```python
from build123d import *

# Parameters (mm, degrees)
SKETCH_3_R               = 7.5
CUT_EXTRUDE_1_DEPTH      = 342.0278581
SKETCH_4_R               = 35
CUT_EXTRUDE_2_DEPTH      = 342.0278581
SWEEP_2_PROFILE_R        = 5.5
CUT_EXTRUDE_4_DEPTH      = 20
PATTERN_CIRCULAR_2_COUNT = 5


with BuildPart() as part:
    # Sketch 1 → Revolve 1 (revolve)
    with BuildSketch(Plane(origin=(0, 0, 0), x_dir=(1, 0, 0), z_dir=(0, 1, 0)), mode=Mode.PRIVATE) as revolve_1_sk:
        Polygon((170, 0), (190, 0), (190, -12), (176, -12), (176, -188), (190, -188), (190, -200), (170, -200), align=None)
    revolve(revolve_1_sk.sketch.rotate(Axis((0, 0, 0), (0, 0, 1)), 180), axis=Axis((0, 0, 0), (0, 0, 1)))

    # Sketch 2 → Revolve 2 (revolve)
    with BuildSketch(Plane(origin=(0, 0, 0), x_dir=(1, 0, 0), z_dir=(0, 1, 0)), mode=Mode.PRIVATE) as revolve_2_sk:
        Polygon((0, -140), (60, -140), (60, -150), (171, -150), (171, -170), (60, -170), (60, -210), (0, -210), align=None)
    revolve(revolve_2_sk.sketch.rotate(Axis((0, 0, 140), (0, 0, 1)), 180), axis=Axis((0, 0, 140), (0, 0, 1)))

    # Sketch 3 → Cut-Extrude 1 (cut, through all)
    with BuildSketch(Plane.XY.offset(210)):
        with Locations(Location((0, 57.15, 0), (0, 0, 18.896417832))):
            Circle(SKETCH_3_R)
        with Locations(Location((-54.35288, 17.660321, 0), (0, 0, 90.896417923))):
            Circle(SKETCH_3_R)
        with Locations(Location((-33.591927, -46.235321, 0), (0, 0, 305.10357978))):
            Circle(SKETCH_3_R)
        with Locations(Location((33.591927, -46.235321, 0), (0, 0, 17.103579776))):
            Circle(SKETCH_3_R)
        with Locations(Location((54.35288, 17.660321, 0), (0, 0, 306.896417429))):
            Circle(SKETCH_3_R)
    extrude(amount=-CUT_EXTRUDE_1_DEPTH, mode=Mode.SUBTRACT)

    # Sketch 4 → Cut-Extrude 2 (cut, through all)
    with BuildSketch(Plane.XY.offset(210)):
        Circle(SKETCH_4_R)
    extrude(amount=-CUT_EXTRUDE_2_DEPTH, mode=Mode.SUBTRACT)

    # Sweep 2: sweep along a curve in space
    with BuildLine() as sweep_2_path:
        Line((94.046, 129.443, 100), (124.876, 171.912, 100))
    # Sweep 2 profile (on start of the path) → Sweep 2 (sweep, cut)
    with BuildSketch(Plane(origin=(94.046, 129.443, 100), x_dir=(0.8092483062128621, -0.5874667470517917, 0), z_dir=(0.5874667470517917, 0.8092483062128621, 0))):
        Circle(SWEEP_2_PROFILE_R)
    sweep(path=sweep_2_path.line, mode=Mode.SUBTRACT)

    # Sketch 13 → Cut-Extrude 4 (cut)
    with BuildSketch(Plane.XY.offset(150)):
        with BuildLine():
            Line((19.985, 80.154), (35.509, 142.42))
            ThreePointArc((35.509, 142.42), (39.332805709, 147.47355651), (45.634, 148.148))
            ThreePointArc((45.634, 148.148), (91.104811943, 125.399590257), (126.78, 89.173))
            ThreePointArc((126.78, 89.173), (128.075469778, 82.982322033), (124.477, 77.781))
            Line((124.477, 77.781), (70.055, 43.775))
            ThreePointArc((70.055, 43.775), (64.394250952, 42.695581589), (59.473, 45.694))
            ThreePointArc((59.473, 45.694), (44.083519984, 60.676348797), (25.08, 70.685))
            ThreePointArc((25.08, 70.685), (20.709688829, 74.438697073), (19.985, 80.154))
        make_face()
    cut_extrude_4 = extrude(amount=CUT_EXTRUDE_4_DEPTH, mode=Mode.SUBTRACT)

    # Pattern Circular 2: Cut-Extrude 4 ×5 about axis
    pattern_circular_2_axis = Axis((0, 0, 0), (0, 0, 1))
    for i in range(1, PATTERN_CIRCULAR_2_COUNT):
        add(cut_extrude_4.rotate(pattern_circular_2_axis, i * 360 / PATTERN_CIRCULAR_2_COUNT), mode=Mode.SUBTRACT)


solid = part.part
```
Part model, mm, in its own coordinate system. A direction names the side the tool comes from. Coordinates: 2 decimals unless noted, no trailing zeros. Order: outer loops, then holes, each group sorted by start corner. A loop starts at its lowest first (then second) coordinate and runs counter-clockwise, first axis right, second up. Notation, with made-up numbers: (71.25, 42.5) -> (129.25, 42.5) arc R21 ccw to (129.25, 76.5) -> close; hole circle Ø1 at (-28.75, 56). An arc over 180 degrees is marked (long way). Put each result on its own line as item: value. Start each with the question number.
(1) Which spindle directions (+Z, -Z, +X, -X, +Y, -Y) get a long thin tool onto all of the face, cutting with end or side? Do faces 4 (the face through (-71.42, -22.89, 159.86)), 5 (the face through (56.93, -18.95, 190.28)). Say none if no direction does.
(2) Band-saw the part on A-A (x = 0). Count the separate pieces of the cut face and the enclosed holes in it, then the cut area to 3 significant figures.
(3) Pin check, flat tips, straight feed: pin 1 Ø8 at (y, z) = (103, 108) entering from -X; pin 2 Ø10 at (x, y) = (150.5, -65.5) entering from -Z; pin 3 Ø6 at (y, z) = (-3.5, 121) entering from -X; pin 4 Ø13.5 at (x, y) = (33.59, -46.24) entering from +Z. Stop position of each tip, or through.
(4) Probe line 1 along Z through (x, y) = (83, 166); line 2 along Y through (x, z) = (11.5, 173); line 3 along Y through (x, z) = (146, 50). List the from-to ranges inside material, lowest first. Write a range as [from, to].
(5) Band-saw the part on B-B (z = 86). Give the cut face in (x, y).
(6) Mould opens along Z. For faces 1 (the face through (-168, 55, 12)), 2 (the face through (12, 62, 150)), 3 (the face through (-64.315, 42.714, 159.86)) say: pulls with the +Z half, pulls with the -Z half, needs draft (parallel to the pull), parting line crosses it, or undercut.
Determined:
1. face 4: +Z, -Z
1. face 5: +Z
2. separate pieces: 4
2. enclosed holes: 0
2. area: 8,550 mm²
3. pin 1: stops at x = -145.52
3. pin 2: stops at z = 150
3. pin 3: stops at x = -176
3. pin 4: passes through
4. line 1: z = [0, 12], [188, 200]
4. line 2: y = [-175.62, -169.61], [-58.89, -33.06], [33.06, 58.89], [169.61, 175.62]
4. line 3: y = [-98.29, -87.09], [87.09, 98.29]
5. outline: circle Ø352 at (0, 0); hole circle Ø340 at (0, 0)
6. face 1: undercut
6. face 2: pulls with the -Z half
6. face 3: needs draft
